Build history of the part. All positions in model axes, mm. A direction names the side the tool comes from. Give positions to 0.01 mm unless a question says otherwise; leave off trailing zeros. Write each loop counter-clockwise with the first axis right and the second up, starting at its lowest first coordinate (ties: lowest second). Pieces come first, ordered by that corner, then holes. Notation, with made-up numbers: (-36.75, 60.5) -> (-18.75, 60.5) arc R21 cw to (-18.75, 99.5) -> close; hole circle Ø6 at (64, 29.5). An arc over 180 degrees is marked (long way). Write item = value, one per line. Start each with the question number.
Q1. Saw through at C-C, the plane y = -5. List the corners of the cut face in (x, z), then the cut area to 3 significant figures.
Q2. Saw through at B-B, the plane z = 4.75. List the corners of the cut face in (x, y), then the cut area to 3 significant figures.
Q3. Drop flat-ended pins along their axis: P1, Ø1.1, axis at x = 79, z = 0, coming from the +Y side; P2, Ø4, axis at x = 94.5, y = 0, coming from the -Z side; P3, Ø4, axis at x = 118, y = 0, coming from the +Z side. Give the stop position or say it passes through.
Q4. Saw through at A-A, the plane x = 38.5. List the corners of the cut face in (y, z), then the cut area to 3 significant figures.
Q5. Wall check: line 1 (X direction, y = -3.5, z = 0.75); line 2 (Z direction, x = 165, y = 1). Give the ranges that are in metal, low to high.
Q6. Tool access for faces 1 (the face through (83, 2.794, 0)), 2 (the face through (83, 0, 2.794)), 3 (the face through (83, 0, -2.794)), 4 (the face through (83, -2.794, 0)), 5 (the face through (-6.157, -1.915, -1.468)): list every direction of +Z, -Z, +X, -X, +Y, -Y with a clear straight run to the whole face (end or side of a thin tool).
Autodesk Inventor part; units mm, degrees
ref_plane "rod_cp_XY" through (0, 0, 0) normal (1, 0, 0) x (0, 0, -1)
ref_plane "rod_cp_YZ" through (0, 0, 0) normal (0, 0, -1) x (0, 1, 0)
ref_plane "rod_cp_ZX" through (0, 0, 0) normal (0, 1, 0) x (1, 0, 0)
sketch "Sketch_1" plane through (0, 0, 0) normal (0, 0, 1) x (1, 0, 0)
  line L0 (184.912, 0) -> (0, 0)
  line L1 (0, 0) -> (0, 2.413)
  arc A0 (1.27, 4.191) -> (0, 2.413) centre (86.3143, -57.8975) ccw
  line L2 (1.27, 4.191) -> (169.0624, 4.191)
  line L3 (169.0624, 4.191) -> (169.0624, 7.22)
  line L4 (169.0624, 7.22) -> (184.912, 7.22)
  line L5 (184.912, 7.22) -> (184.912, 0)
  line L6 (184.912, 0) -> (0, 0)
revolve "Revolution1" add sketch "Sketch_1" angle 360 about axis through (184.912, 0, 0) along (1, 0, 0)
sketch "Sketch_3" plane through (0, 0, 0) normal (0, 0, 1) x (1, 0, 0)
  line L0 (0, 0) -> (-12.7, 0)
  line L1 (-12.7, 0) -> (-12.7, 1.9406)
  line L2 (-12.7, 1.9406) -> (-12.2276, 2.413)
  line L3 (-12.2276, 2.413) -> (0, 2.413)
  line L4 (0, 2.413) -> (0, 0)
  line L5 (0, 0) -> (-12.7, 0)
revolve "Revolution2" add sketch "Sketch_3" angle 360 about axis through (0, 0, 0) along (1, 0, 0)
thread "Thread1"
sketch "Sketch_31" plane through (0, 0, 0) normal (1, 0, 0) x (0, 0, -1)
  line L0 (-5.588, 5.588) -> (-5.588, -5.588)
  line L1 (-5.588, -5.588) -> (5.588, -5.588)
  line L2 (5.588, -5.588) -> (5.588, 5.588)
  line L3 (5.588, 5.588) -> (-5.588, 5.588)
  line L4 (-2.794, 1.778) -> (-2.794, -1.778)
  arc A0 (-2.794, -1.778) -> (-1.778, -2.794) centre (-1.778, -1.778) ccw
  line L5 (-1.778, -2.794) -> (1.778, -2.794)
  arc A1 (1.778, -2.794) -> (2.794, -1.778) centre (1.778, -1.778) ccw
  line L6 (2.794, -1.778) -> (2.794, 1.778)
  arc A2 (2.794, 1.778) -> (1.778, 2.794) centre (1.778, 1.778) ccw
  line L7 (1.778, 2.794) -> (-1.778, 2.794)
  arc A3 (-1.778, 2.794) -> (-2.794, 1.778) centre (-1.778, 1.778) ccw
extrude "Extrusion1" cut sketch "Sketch_31" along normal mid plane 338.1248
sketch "Sketch_30" plane through (0, 0, 0) normal (0, 0, 1) x (1, 0, 0)
  line L0 (0, 0) -> (-0.254, 0)
  line L1 (-0.254, 2.413) -> (-0.254, 2.159)
  line L2 (-0.254, 2.159) -> (0, 2.159)
  line L3 (0, 2.159) -> (0, 2.413)
  line L4 (0, 2.413) -> (-0.254, 2.413)
revolve "Revolution3" cut sketch "Sketch_30" angle 360 about axis through (0, 0, 0) along (1, 0, 0)
ref_plane "rod_cp_XY" through (0, 0, 0) normal (1, 0, 0) x (0, 0, -1)
ref_plane "rod_cp_YZ" through (0, 0, 0) normal (0, 0, -1) x (0, 1, 0)
ref_plane "rod_cp_ZX" through (0, 0, 0) normal (0, 1, 0) x (1, 0, 0)
ref_plane "to_rod_clevis_XY" through (-12.7, 0, 0) normal (1, 0, 0) x (0, 0, -1)
ref_plane "to_rod_clevis_YZ" through (-12.7, 0, 0) normal (0, 0, -1) x (0, 1, 0)
ref_plane "to_rod_clevis_ZX" through (-12.7, 0, 0) normal (0, 1, 0) x (1, 0, 0)
ref_plane "rl22_XY" through (0, 0, 0) normal (1, 0, 0) x (0, 0, -1)
ref_plane "rl22_YZ" through (0, 0, 0) normal (0, 0, -1) x (0, 1, 0)
ref_plane "rl22_ZX" through (0, 0, 0) normal (0, 1, 0) x (1, 0, 0)
ref_plane "rl1_XY" through (-12.7, 0, 0) normal (1, 0, 0) x (0, 0, -1)
ref_plane "rl1_YZ" through (-12.7, 0, 0) normal (0, 0, -1) x (0, 1, 0)
ref_plane "rl1_ZX" through (-12.7, 0, 0) normal (0, 1, 0) x (1, 0, 0)
ref_plane "thd1_XY" through (-12.7, 2.413, 0) normal (1, 0, 0) x (0, 0, -1)
ref_plane "thd1_YZ" through (-12.7, 2.413, 0) normal (0, 0, -1) x (0, 1, 0)
ref_plane "thd1_ZX" through (-12.7, 2.413, 0) normal (0, 1, 0) x (1, 0, 0)
ref_plane "thd2_XY" through (-12.7, -2.413, 0) normal (1, 0, 0) x (0, 0, -1)
ref_plane "thd2_YZ" through (-12.7, -2.413, 0) normal (0, 0, -1) x (0, 1, 0)
ref_plane "thd2_ZX" through (-12.7, -2.413, 0) normal (0, 1, 0) x (1, 0, 0)
ref_plane "dia1_XY" through (0, 2.794, 0) normal (1, 0, 0) x (0, 0, -1)
ref_plane "dia1_YZ" through (0, 2.794, 0) normal (0, 0, -1) x (0, 1, 0)
ref_plane "dia1_ZX" through (0, 2.794, 0) normal (0, 1, 0) x (1, 0, 0)
ref_plane "dia2_XY" through (0, -2.794, 0) normal (1, 0, 0) x (0, 0, -1)
ref_plane "dia2_YZ" through (0, -2.794, 0) normal (0, 0, -1) x (0, 1, 0)
ref_plane "dia2_ZX" through (0, -2.794, 0) normal (0, 1, 0) x (1, 0, 0)
ref_plane "stroke11_XY" through (0, 0, 0) normal (1, 0, 0) x (0, 0, -1)
ref_plane "stroke11_YZ" through (0, 0, 0) normal (0, 0, -1) x (0, 1, 0)
ref_plane "stroke11_ZX" through (0, 0, 0) normal (0, 1, 0) x (1, 0, 0)
ref_plane "h1_XY" through (3.175, 0, 0) normal (0, 0, 1) x (1, 0, 0)
ref_plane "h1_YZ" through (3.175, 0, 0) normal (1, 0, 0) x (0, 1, 0)
ref_plane "h1_ZX" through (3.175, 0, 0) normal (0, 1, 0) x (0, 0, 1)
ref_plane "h2_XY" through (0, 0, 0) normal (0, 0, 1) x (1, 0, 0)
ref_plane "h2_YZ" through (0, 0, 0) normal (1, 0, 0) x (0, 1, 0)
ref_plane "h2_ZX" through (0, 0, 0) normal (0, 1, 0) x (0, 0, 1)
ref_plane "h3_XY" through (0, 0, 0) normal (0, 0, 1) x (1, 0, 0)
ref_plane "h3_YZ" through (0, 0, 0) normal (1, 0, 0) x (0, 1, 0)
ref_plane "h3_ZX" through (0, 0, 0) normal (0, 1, 0) x (0, 0, 1)
ref_plane "rl2_XY" through (0, 0, 0) normal (1, 0, 0) x (0, 0, -1)
ref_plane "rl2_YZ" through (0, 0, 0) normal (0, 0, -1) x (0, 1, 0)
ref_plane "rl2_ZX" through (0, 0, 0) normal (0, 1, 0) x (1, 0, 0)
ref_plane "stroke1_XY" through (0, 0, 0) normal (1, 0, 0) x (0, 0, -1)
ref_plane "stroke1_YZ" through (0, 0, 0) normal (0, 0, -1) x (0, 1, 0)
ref_plane "stroke1_ZX" through (0, 0, 0) normal (0, 1, 0) x (1, 0, 0)
ref_plane "dia12_XY" through (0, 0, 7.8105) normal (1, 0, 0) x (0, 0, -1)
ref_plane "dia12_YZ" through (0, 0, 7.8105) normal (0, 0, -1) x (0, 1, 0)
ref_plane "dia12_ZX" through (0, 0, 7.8105) normal (0, 1, 0) x (1, 0, 0)
ref_plane "dia22_XY" through (0, 0, -7.8105) normal (1, 0, 0) x (0, 0, -1)
ref_plane "dia22_YZ" through (0, 0, -7.8105) normal (0, 0, -1) x (0, 1, 0)
ref_plane "dia22_ZX" through (0, 0, -7.8105) normal (0, 1, 0) x (1, 0, 0)
ref_plane "stroke1bf_XY" through (0, 0, 0) normal (1, 0, 0) x (0, 0, -1)
ref_plane "stroke1bf_YZ" through (0, 0, 0) normal (0, 0, -1) x (0, 1, 0)
ref_plane "stroke1bf_ZX" through (0, 0, 0) normal (0, 1, 0) x (1, 0, 0)
properties part number "025.5-D_NR_rod"
Report:
q1.outline = (169.06, -5.21) -> (184.91, -5.21) -> (184.91, 5.21) -> (169.06, 5.21) -> close
q1.area = 165 mm2
q2.outline = (169.06, -5.44) -> (184.91, -5.44) -> (184.91, 5.44) -> (169.06, 5.44) -> close
q2.area = 172 mm2
q3.P1 = 2.79
q3.P2 = -2.79
q3.P3 = 2.79
q4.outline = (-2.79, -1.78) arc R1.02 ccw to (-1.78, -2.79) -> (1.78, -2.79) arc R1.02 ccw to (2.79, -1.78) -> (2.79, 1.78) arc R1.02 ccw to (1.78, 2.79) -> (-1.78, 2.79) arc R1.02 ccw to (-2.79, 1.78) -> close
q4.area = 30.3 mm2
q5.line_1 = 169.06 to 184.91
q5.line_2 = -2.79 to 2.79
q6.face_1 = +Z, -Z, -X, +Y
q6.face_2 = +Z, -X, +Y, -Y
q6.face_3 = -Z, -X, +Y, -Y
q6.face_4 = +Z, -Z, -X, -Y
q6.face_5 = -X
